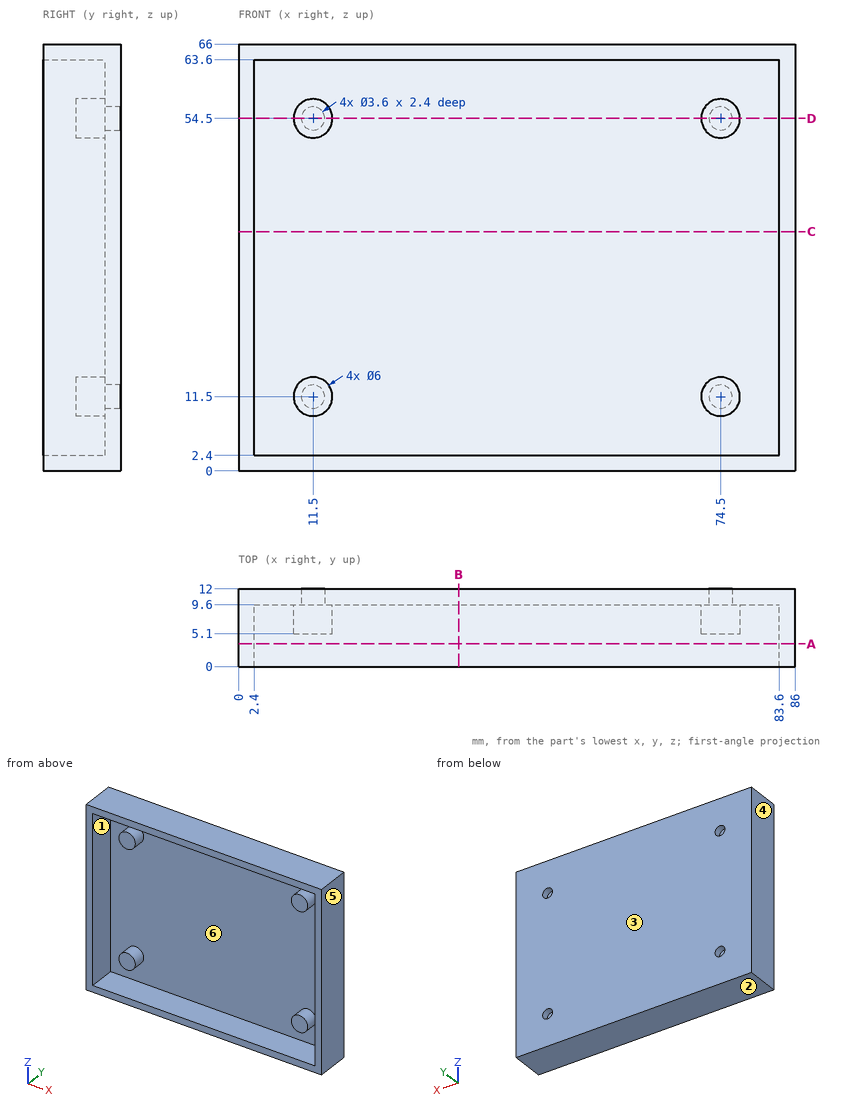
Part print with two shaded views. Sizes in mm from the minimum x, y, z corner. A direction names the side the tool comes from. Coordinates: 2 decimals unless noted, no trailing zeros. Loops run counter-clockwise (first coordinate to the right, second up) from the corner with the lowest first, then second, coordinate; pieces in that order, holes last. Notation, with made-up numbers: M 22,49 L 44,49 A34 ccw 44,81 Z; hole C 30,-12 d5. An arc over 180 degrees is marked long. Use CSV: the item, a comma, the result in double quotes. Start each with the question number.
1. Probe probe 1 along Z at (x, y) = (74.5, 10.5); probe 2 along X at (y, z) = (10.5, 54.5); probe 3 along X at (y, z) = (7, 37.5). List the from-to ranges inside material, lowest first. Write a range as [from, to].
2. Band-saw the part on D-D, the plane z = 54.5. List the corners of the cut face in (x, y), then the cut area to 3 significant figures.
3. Band-saw the part on B-B, the plane x = 34. List the corners of the cut face in (y, z), then the cut area to 3 significant figures.
4. Flat gauge pins, fed straight in: pin 1 (4 mm diameter, centred on x = 11.5, z = 54.5, fed in from -Y); pin 2 (1.8 mm diameter, centred on x = 11, z = 55, fed in from +Y). Where does each tip first touch, or does it go through?
5. Tool access for the marked faces 1 and 2: list every direction of +Z, -Z, +X, -X, +Y, -Y with a clear straight run to the whole face (end or side of a thin tool).
6. Band-saw the part on C-C, the plane z = 37. List the corners of the cut face in (x, y), then the cut area to 3 significant figures.
7. Band-saw the part on A-A, the plane y = 3.5. List the corners of the cut face in (x, z), then the cut area to 3 significant figures.
8. Two-plate mould, pull along X, no slides. Class the marked faces 3, 4, 5 and 6: pulls with the +X half, pulls with the -X half, needs draft (parallel to the pull), parting line crosses it, or undercut.
Entries:
1,probe 1,"z = [0, 9.7], [13.3, 52.7], [56.3, 66]"
1,probe 2,"x = [0, 9.7], [13.3, 72.7], [76.3, 86]"
1,probe 3,"x = [0, 2.4], [83.6, 86]"
2,outline,"M 0,0 L 2.4,0 L 2.4,9.6 L 8.5,9.6 L 8.5,5.1 L 14.5,5.1 L 14.5,9.6 L 71.5,9.6 L 71.5,5.1 L 77.5,5.1 L 77.5,9.6 L 83.6,9.6 L 83.6,0 L 86,0 L 86,12 L 76.3,12 L 76.3,9.6 L 72.7,9.6 L 72.7,12 L 13.3,12 L 13.3,9.6 L 9.7,9.6 L 9.7,12 L 0,12 Z"
2,area,"289 mm2"
3,outline,"M 0,0 L 12,0 L 12,66 L 0,66 L 0,63.6 L 9.6,63.6 L 9.6,2.4 L 0,2.4 Z"
3,area,"204 mm2"
4,pin 1,"stops at y = 5.1"
4,pin 2,"stops at y = 9.6"
5,face 1,"-Y"
5,face 2,"-Z, +X, -X, +Y, -Y"
6,outline,"M 0,0 L 2.4,0 L 2.4,9.6 L 83.6,9.6 L 83.6,0 L 86,0 L 86,12 L 0,12 Z"
6,area,"252 mm2"
7,outline,"M 0,0 L 86,0 L 86,66 L 0,66 Z; hole M 2.4,2.4 L 83.6,2.4 L 83.6,63.6 L 2.4,63.6 Z"
7,area,"707 mm2"
8,face 3,"needs draft"
8,face 4,"pulls with the -X half"
8,face 5,"pulls with the +X half"
8,face 6,"undercut"
